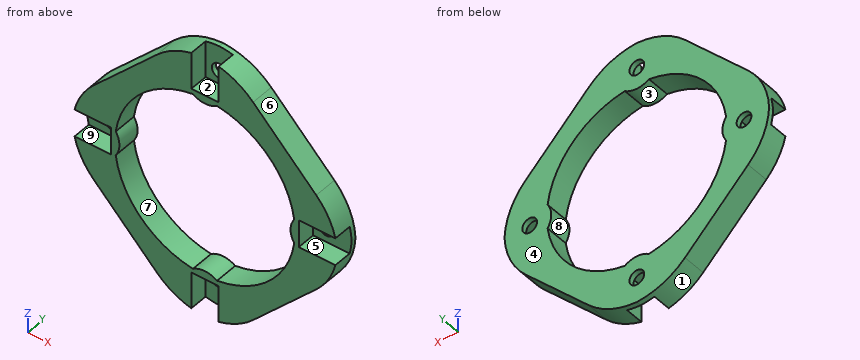
from build123d import *

# Parameters (mm, degrees)
SKETCH1_R           = 75
SKETCH1_R_2         = 50
BOSS_EXTRUDE1_DEPTH = 13
SKETCH2_R           = 4.1
CUT_EXTRUDE1_DEPTH  = 107.85972113
SKETCH8_R           = 12
SKETCH8_R_2         = 4.1
BOSS_EXTRUDE4_DEPTH = 13
SKETCH3_W           = 15.2
SKETCH3_H           = 40
SKETCH3_W_2         = 40
SKETCH3_H_2         = 15.2
CUT_EXTRUDE2_DEPTH  = 10.2
BOSS_EXTRUDE2_DEPTH = 13
FILLET1_R           = 30
SKETCH7_OUTSIDE_W   = 194.506
SKETCH7_OUTSIDE_H   = 194.506
CUT_EXTRUDE4_DEPTH  = 107.85972113
FILLET3_R           = 40


with BuildPart() as part:
    # Sketch1 → Boss-Extrude1 (new body)
    with BuildSketch(Plane(origin=(0, 0, 0), x_dir=(1, 0, 0), z_dir=(0, 1, 0))):
        with Locations(Location((0, 0, 0), (0, 0, 90))):
            Circle(SKETCH1_R)
        with Locations(Location((0, 0, 0), (0, 0, 90))):
            Circle(SKETCH1_R_2, mode=Mode.SUBTRACT)
    extrude(amount=BOSS_EXTRUDE1_DEPTH)

    # Sketch2 → Cut-Extrude1 (cut, through all)
    with BuildSketch(Plane(origin=(0, 13, 0), x_dir=(1, 0, 0), z_dir=(0, 1, 0))):
        with Locations(Location((0, 59.5, 0), (0, 0, 270))):
            Circle(SKETCH2_R)
        with Locations(Location((59.5, 0, 0), (0, 0, 270))):
            Circle(SKETCH2_R)
        with Locations(Location((0, -59.5, 0), (0, 0, 270))):
            Circle(SKETCH2_R)
        with Locations(Location((-59.5, 0, 0), (0, 0, 270))):
            Circle(SKETCH2_R)
    extrude(amount=-CUT_EXTRUDE1_DEPTH, mode=Mode.SUBTRACT)

    # Sketch8 → Boss-Extrude4 (add)
    # profile 1 of 4: a face of its own
    with BuildSketch(Plane(origin=(0, 13, 0), x_dir=(1, 0, 0), z_dir=(0, 1, 0))):
        with Locations((59.5, 0)):
            Circle(SKETCH8_R)
        with Locations(Location((59.5, 0, 0), (0, 0, 270))):
            Circle(SKETCH8_R_2, mode=Mode.SUBTRACT)
    # profile 2 of 4: a face of its own
    with BuildSketch(Plane(origin=(0, 13, 0), x_dir=(1, 0, 0), z_dir=(0, 1, 0))):
        with Locations((0, -59.5)):
            Circle(SKETCH8_R)
        with Locations(Location((0, -59.5, 0), (0, 0, 270))):
            Circle(SKETCH8_R_2, mode=Mode.SUBTRACT)
    # profile 3 of 4: a face of its own
    with BuildSketch(Plane(origin=(0, 13, 0), x_dir=(1, 0, 0), z_dir=(0, 1, 0))):
        with Locations((-59.5, 0)):
            Circle(SKETCH8_R)
        with Locations(Location((-59.5, 0, 0), (0, 0, 270))):
            Circle(SKETCH8_R_2, mode=Mode.SUBTRACT)
    # profile 4 of 4: a face of its own
    with BuildSketch(Plane(origin=(0, 13, 0), x_dir=(1, 0, 0), z_dir=(0, 1, 0))):
        with Locations((0, 59.5)):
            Circle(SKETCH8_R)
        with Locations(Location((0, 59.5, 0), (0, 0, 270))):
            Circle(SKETCH8_R_2, mode=Mode.SUBTRACT)
    extrude(amount=-BOSS_EXTRUDE4_DEPTH)

    # Sketch3 → Cut-Extrude2 (cut)
    with BuildSketch(Plane.XZ):
        with Locations((0, 72.1)):
            Rectangle(SKETCH3_W, SKETCH3_H)
        with Locations((72.1, 0)):
            Rectangle(SKETCH3_W_2, SKETCH3_H_2)
        with Locations((0, -72.1)):
            Rectangle(SKETCH3_W, SKETCH3_H)
        with Locations((-72.1, 0)):
            Rectangle(SKETCH3_W_2, SKETCH3_H_2)
    extrude(amount=-CUT_EXTRUDE2_DEPTH, mode=Mode.SUBTRACT)

    # Sketch4 → Boss-Extrude2 (add)
    with BuildSketch(Plane(origin=(0, 13, 0), x_dir=(1, 0, 0), z_dir=(0, 1, 0))):
        Polygon((-40.658639918, -65.40737726), (-65.40737726, -40.658639918), (-63.943497033, -39.194759691), (-39.194759691, -63.943497033), align=None)
    extrude(amount=-BOSS_EXTRUDE2_DEPTH)

    # Fillet1
    # the kernel refuses this fillet: 30 mm, written as the material it adds along each edge
    with BuildSketch(Plane(origin=(-63.943497033, 13, 39.194759691), x_dir=(-0.47318102872743373, 0, -0.8809652172773041), z_dir=(0, -1, 0))) as fillet1_piece_1:
        with BuildLine():
            CenterArc((10.253688675, -29.951285387), FILLET1_R, 93.265618259, 17.938271436)
            Line((-0.596947211, -1.982307914), (-0.813959928, -1.422928365))
            ThreePointArc((-0.813959928, -1.422928365), (-0.872989201, -0.818145778), (-0.574515596, 0.173008179))
            Line((-0.574515596, 0.173008179), (0.034178962, 0.599025708))
            ThreePointArc((0.034178962, 0.599025708), (4.272370281, 0.478213468), (8.5105616, 0.599025708))
            Line((8.5105616, 0.599025708), (8.544740562, 0))
        make_face()
    extrude(amount=13)
    with BuildSketch(Plane(origin=(-39.194759691, 13, 63.943497033), x_dir=(0.8809652172773019, 0, 0.47318102872743756), z_dir=(0, -1, 0))) as fillet1_piece_2:
        with BuildLine():
            CenterArc((10.253688675, 29.951285387), FILLET1_R, 248.796110305, 17.938271436)
            Line((-0.596947211, 1.982307914), (-0.813959928, 1.422928365))
            ThreePointArc((-0.813959928, 1.422928365), (-0.872989201, 0.818145778), (-0.574515596, -0.173008179))
            Line((-0.574515596, -0.173008179), (0.034178962, -0.599025708))
            ThreePointArc((0.034178962, -0.599025708), (4.272370281, -0.478213468), (8.5105616, -0.599025708))
            Line((8.5105616, -0.599025708), (8.544740562, 0))
        make_face()
    extrude(amount=13)

    # Sketch7 outside → Cut-Extrude4 (cut, through all)
    with BuildSketch(Plane(origin=(0, 13, 0), x_dir=(1, 0, 0), z_dir=(0, 1, 0))):
        Rectangle(SKETCH7_OUTSIDE_W, SKETCH7_OUTSIDE_H)
        Polygon((73.484692283, -15), (15, -73.484692283), (-15, -73.484692283), (-73.484692283, -15), (-73.484692283, 15), (-15, 73.484692283), (15, 73.484692283), (73.484692283, 15), align=None, mode=Mode.SUBTRACT)
    extrude(amount=-CUT_EXTRUDE4_DEPTH, mode=Mode.SUBTRACT)

    # Fillet3
    # the kernel refuses this fillet: 40 mm, written as the material it takes off along each edge
    with BuildSketch(Plane(origin=(15, 54.421356237, 73.484692283), x_dir=(-1, 0, 0), z_dir=(0, -1, 0)), Plane(origin=(73.484692283, 54.421356237, 15), x_dir=(-0.7071067811865474, 0, 0.7071067811865476), z_dir=(0, -1, 0))) as fillet3_piece_1:
        with BuildLine():
            CenterArc((FILLET3_R * 0.414213562373, FILLET3_R), FILLET3_R, 225, 45)
            Line((-FILLET3_R * 0.292893218813, FILLET3_R * 0.292893218813), (0, 0))
            Line((0, 0), (FILLET3_R * 0.414213562373, 0))
        make_face()
    extrude(amount=95.842712475, mode=Mode.SUBTRACT)
    with BuildSketch(Plane(origin=(-15, 54.421356237, 73.484692283), x_dir=(1, 0, 0), z_dir=(0, -1, 0)), Plane(origin=(-73.484692283, 54.421356237, 15), x_dir=(0.7071067811865477, 0, 0.7071067811865472), z_dir=(0, -1, 0)), Plane(origin=(-73.484692283, 54.421356237, -15), x_dir=(0, 0, 1), z_dir=(0, -1, 0)), Plane(origin=(-15, 54.421356237, -73.484692283), x_dir=(-0.7071067811865472, 0, 0.7071067811865477), z_dir=(0, -1, 0)), Plane(origin=(15, 54.421356237, -73.484692283), x_dir=(-1, 0, 0), z_dir=(0, -1, 0)), Plane(origin=(73.484692283, 54.421356237, -15), x_dir=(-0.7071067811865477, 0, -0.7071067811865472), z_dir=(0, -1, 0))) as fillet3_piece_2:
        with BuildLine():
            CenterArc((FILLET3_R * 0.414213562373, -FILLET3_R), FILLET3_R, 90, 45)
            Line((-FILLET3_R * 0.292893218813, -FILLET3_R * 0.292893218813), (0, 0))
            Line((0, 0), (FILLET3_R * 0.414213562373, 0))
        make_face()
    extrude(amount=95.842712475, mode=Mode.SUBTRACT)


solid = part.part
The listing builds one solid part. Answer for the finished solid, in the listing's coordinates (mm). Face numbers are marked on the shaded views. A direction names the side the tool comes from. Round coordinates to 2 decimals unless told otherwise and drop trailing zeros. Order: outer loops, then holes, each group sorted by start corner. A loop starts at its lowest first (then second) coordinate and runs counter-clockwise, first axis right, second up. Notation, with made-up numbers: (31, 28.25) - (77, 28.25) arc R36 ccw to (77, 62.25) - close; hole circle Ø4 at (-11, 69.25). An arc over 180 degrees is marked (long way). Write item = value, one per line. Start each with the question number.
1) Section D-D, the plane z = -58 is taken. Write down the section's boundary in (x, y), plus the area to 3 significant figures.
2) Given pin 1 (3 mm diameter, centred on y = 5, z = 61, fed in from +X); pin 2 (6.5 mm diameter, centred on x = -59.5, z = 0, fed in from +Y); pin 3 (1 mm diameter, centred on y = 6.5, z = -46.5, fed in from +X); pin 4 (5 mm diameter, centred on y = 6, z = 65.5, fed in from -X), each flat-ended and moving along its own axis, determine where each tip first touches the part or whether it passes through.
3) For a pull along X with two mould halves and no side action, classify the marked faces 6, 7, 8 and 9 as released by +X, released by -X, zero draft, split by the parting line, or undercut.
4) Section C-C, the plane z = 45 is taken. Write down the section's boundary in (x, y), plus the area to 3 significant figures.
5) For the marked faces 1, 2, 3, 4 and 5, determine the directions among +Z, -Z, +X, -X, +Y, -Y from which every point of the face is accessible in a straight line to the end or side of a thin tool.
6) Straight lines are drawn through the part: L1, parallel to X at y = 1.75, z = -57; L2, parallel to X at y = 11.9, z = -59.5; L3, parallel to Y at x = -7, z = 53.5. For each, find the intervals that lie inside material, in ascending order.
7) Section B-B, the plane x = -59.5 is taken. Write down the section's boundary in (y, z), plus the area to 3 significant figures.
8) Section A-A, the plane z = -13.5 is taken. Write down the section's boundary in (x, y).
Results list:
q1.outline = (-30.48, 0) - (-7.6, 0) - (-7.6, 10.2) - (-3.82, 10.2) - (-3.82, 13) - (-30.48, 13) - close; (3.82, 10.2) - (7.6, 10.2) - (7.6, 0) - (30.48, 0) - (30.48, 13) - (3.82, 13) - close
q1.area = 616 mm^2
q2.pin_1 = 28.98
q2.pin_2 = through
q2.pin_3 = 42.48
q2.pin_4 = -25.43
q3.face_6 = released by +X
q3.face_7 = undercut
q3.face_8 = undercut
q3.face_9 = zero draft
q4.outline = (-43.48, 0) - (-21.79, 0) - (-21.79, 13) - (-43.48, 13) - close; (21.79, 0) - (43.48, 0) - (43.48, 13) - (21.79, 13) - close
q4.area = 564 mm^2
q5.face_1 = -Z, -X, +Y, -Y
q5.face_2 = +Z, -Y
q5.face_3 = +Y, -Y
q5.face_4 = +Z, -Z, +X, -X, +Y
q5.face_5 = +X, -Y
q6.L1 = -31.48 to -7.6, 7.6 to 31.48
q6.L2 = -28.98 to -4.1, 4.1 to 28.98
q6.L3 = 10.2 to 13
q7.outline = (0, -28.98) - (13, -28.98) - (13, -4.1) - (10.2, -4.1) - (10.2, -7.6) - (0, -7.6) - close; (0, 7.6) - (10.2, 7.6) - (10.2, 4.1) - (13, 4.1) - (13, 28.98) - (0, 28.98) - close
q7.area = 576 mm^2
q8.outline = (-70.54, 0) - (-48.14, 0) - (-48.14, 13) - (-70.54, 13) - close; (48.14, 0) - (70.54, 0) - (70.54, 13) - (48.14, 13) - close
